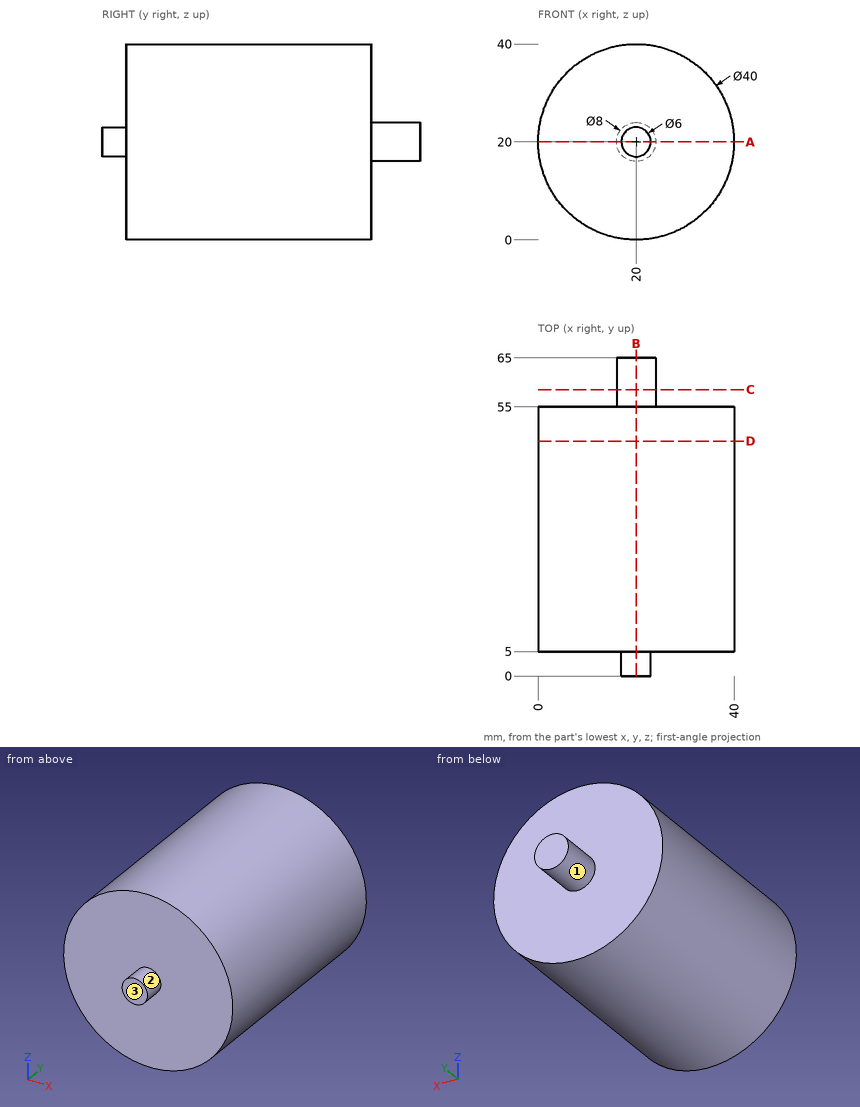
The figure shows three views and two pictorial views of one solid part (mm, origin at its lowest corner). Answer the questions. A direction names the side the tool comes from. Round coordinates to 2 decimals unless told otherwise and drop trailing zeros. Write each loop counter-clockwise with the first axis right and the second up, starting at its lowest first coordinate (ties: lowest second). Pieces come first, ordered by that corner, then holes. Notation, with made-up numbers: (-18, 89) - (-13, 89) arc R19 ccw to (-13, 123) - close; hole circle Ø5 at (54.5, 89.5). An arc over 180 degrees is marked (long way). One line per question, with ' | ' between items. Start each with the question number.
1. For the marked faces 1, 2 and 3, determine the directions among +Z, -Z, +X, -X, +Y, -Y from which every point of the face is accessible in a straight line to the end or side of a thin tool.
2. Section D-D (y = 48) is taken. Determine the outline of the cut face in (x, z).
3. Each of these flat-tipped pins is pushed along its axis until it touches: pin 1 (2 mm diameter, centred on x = 30, y = 12.5, fed in from +Z); pin 2 (6 mm diameter, centred on y = 40.5, z = 27.5, fed in from -X); pin 3 (8 mm diameter, centred on x = 16.5, z = 7.5, fed in from +Y). Where does it stop, or does it pass through?
4. Section C-C (y = 58.5) is taken. Determine the outline of the cut face in (x, z).
5. Section B-B (x = 20) is taken. Determine the outline of the cut face in (y, z).
6. Find the intervals of material crossed by probe 1 along X at (y, z) = (7, 20); probe 2 along Y at (x, z) = (19, 2); probe 3 along Z at (x, y) = (25.5, 50.5), in increasing order. Write a range as [from, to].
7. Section A-A (z = 20) is taken. Determine the outline of the cut face in (x, y), and give its area (3 significant figures).
Filled in:
1) face 1: +Y | face 2: -Y | face 3: +Z, -Z, +X, -X, -Y
2) outline: circle Ø40 at (20, 20)
3) pin 1: z = 37.86 | pin 2: x = 0.51 | pin 3: y = 55
4) outline: circle Ø8 at (20, 20)
5) outline: (0, 17) - (5, 17) - (5, 0) - (55, 0) - (55, 16) - (65, 16) - (65, 24) - (55, 24) - (55, 40) - (5, 40) - (5, 23) - (0, 23) - close
6) probe 1: [0, 40] | probe 2: [5, 55] | probe 3: [0.77, 39.23]
7) outline: (0, 5) - (17, 5) - (17, 0) - (23, 0) - (23, 5) - (40, 5) - (40, 55) - (24, 55) - (24, 65) - (16, 65) - (16, 55) - (0, 55) - close | area: 2,110 mm²
